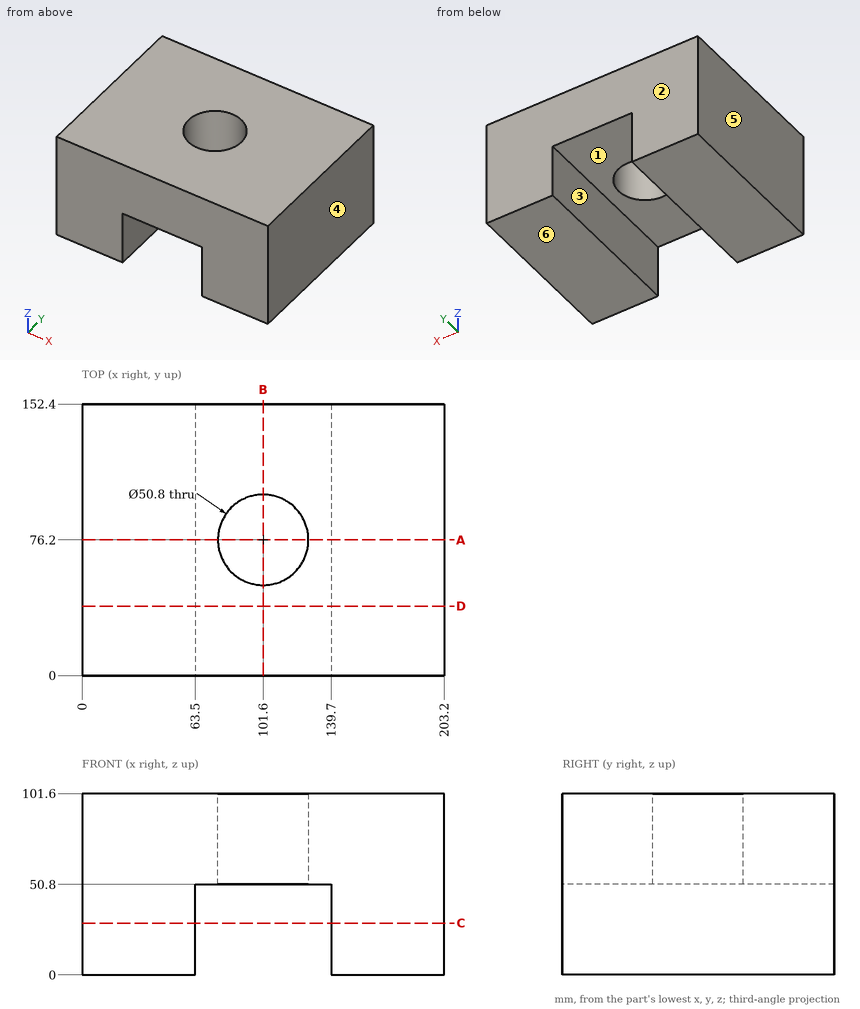
Could you check a few things on this drawing? It's one solid part, dimensions in mm from its lowest x, y, z. A direction names the side the tool comes from. Give positions to 0.01 mm unless a question says otherwise; leave off trailing zeros. Loops run counter-clockwise (first coordinate to the right, second up) from the corner with the lowest first, then second, coordinate; pieces in that order, holes last. Notation, with made-up numbers: M 58,42 L 109,42 A11 cw 109,62 Z; hole C 21.5,-7 d11. An arc over 180 degrees is marked long. Return JSON: item names as keys, results as strings.
Item 1: Imagine slicing it at C-C on z = 29. List the corners of the cut face in (x, y) for me, then the cut area to 3 significant figures.
A:
{"outline": "M 0,0 L 63.5,0 L 63.5,152.4 L 0,152.4 Z; M 139.7,0 L 203.2,0 L 203.2,152.4 L 139.7,152.4 Z", "area": "19,400 mm^2"}
Item 2: Imagine slicing it at B-B on x = 101.6. List the corners of the cut face in (y, z) for me.
A:
{"outline": "M 0,50.8 L 50.8,50.8 L 50.8,101.6 L 0,101.6 Z; M 101.6,50.8 L 152.4,50.8 L 152.4,101.6 L 101.6,101.6 Z"}
Item 3: Imagine slicing it at D-D on y = 39. List the corners of the cut face in (x, z) for me.
A:
{"outline": "M 0,0 L 63.5,0 L 63.5,50.8 L 139.7,50.8 L 139.7,0 L 203.2,0 L 203.2,101.6 L 0,101.6 Z"}
Item 4: Please list where these lines run through material, in increasing order: line 1 (X direction, y = 63.5, z = 12); line 2 (X direction, y = 76, z = 65); line 3 (Y direction, x = 101.6, z = 87).
A:
{"line 1": "x = 0 to 63.5, 139.7 to 203.2", "line 2": "x = 0 to 76.2, 127 to 203.2", "line 3": "y = 0 to 50.8, 101.6 to 152.4"}
Item 5: On a 3-axis mill with a long thin cutter (end or side, diameter ignored), from which of +Z, -Z, +X, -X, +Y, -Y can I reach the whole of each face in a straight line? I mean the marked faces 1 and 2. Say none if no direction works.
A:
{"face 1": "-Z, +Y, -Y", "face 2": "+Z, -Z, +X, -X, +Y"}
Item 6: Thinking about a two-plate mould opening in X: for the marked faces 3, 4, 5 and 6, which applies, released by +X, released by -X, zero draft, split by the parting line, or undercut?
A:
{"face 3": "undercut", "face 4": "released by +X", "face 5": "released by -X", "face 6": "zero draft"}
Item 7: Imagine slicing it at A-A on y = 76.2. List the corners of the cut face in (x, z) for me, then the cut area to 3 significant figures.
A:
{"outline": "M 0,0 L 63.5,0 L 63.5,50.8 L 76.2,50.8 L 76.2,101.6 L 0,101.6 Z; M 127,50.8 L 139.7,50.8 L 139.7,0 L 203.2,0 L 203.2,101.6 L 127,101.6 Z", "area": "14,200 mm^2"}
Item 8: I'm going to push flat-ended pins straight in: pin 1 Ø8 at (x, z) = (112, 84) entering from -Y; pin 2 Ø23 at (x, y) = (112, 97.5) entering from -Z. Where does each tip first touch, or does it pass through?
A:
{"pin 1": "stops at y = 0", "pin 2": "stops at z = 50.8"}
